Build history of the part. All positions in model axes, mm. Face numbers are marked on the shaded views. A direction names the side the tool comes from. Coordinates: 2 decimals unless noted, no trailing zeros. Loops run counter-clockwise (first coordinate to the right, second up) from the corner with the lowest first, then second, coordinate; pieces in that order, holes last.
(1) Slice it at D-D (x = -82.5). Give the cut face in (y, z).
(2) Flat gauge pins, fed straight in: P1, Ø6, axis at x = 1.5, z = -9.5, coming from the -Y side; P2, Ø1.5, axis at y = -232.5, z = -66.5, coming from the -X side; P3, Ø0.9, axis at y = -221.5, z = -13.5, coming from the +X side. Where does each tip first touch, or does it go through?
(3) Slice it at B-B (z = -96). Give the cut face in (x, y).
(4) Two-plate mould, pull along X, no slides. Class the marked faces 1, 2 and 3: pulls with the +X half, pulls with the -X half, needs draft (parallel to the pull), parting line crosses it, or undercut.
(5) Slice it at A-A (z = -12). Give the cut face in (x, y), and give its area (3 significant figures).
(6) Tool access for the marked faces 4 and 5: list every direction of +Z, -Z, +X, -X, +Y, -Y with a clear straight run to the whole face (end or side of a thin tool).
(7) Wall check: L1, parallel to Z at x = 0, y = -221; L2, parallel to X at y = -247, z = -1; L3, parallel to Y at x = 0, z = -1. Give the ranges that are in metal, low to high.
(8) Slice it at C-C (y = 102.5). Give the cut face in (x, z).
Autodesk Inventor part; units mm, degrees
ref_plane "Work Plane1" through (30, -275.6, -108.75) normal (1, 0, 0) x (0, 0, -1)
ref_plane "Work Plane2" through (0, -278.6, 0) normal (1, 0, 0) x (0, 0, -1)
ref_plane "Work Plane3" through (0, -275.6, 0) normal (1, 0, 0) x (0, 0, -1)
sketch "Sketch1" plane through (0, 0, 0) normal (0, 0, 1) x (1, 0, 0)
  line L0 (-100, 150) -> (100, 150)
  line L1 (100, 150) -> (100, -150)
  line L2 (-100, -150) -> (-100, 150)
  line L3 (-100, 150) -> (100, -150) construction
  line L4 (100, 150) -> (-100, -150) construction
  line L5 (100, -150) -> (36.4382, -213.5618)
  line L6 (-35.3571, -283.1536) -> (-35.3571, -323.1554)
  line L7 (-35.3571, -323.1554) -> (21.2114, -379.7239)
  line L8 (35.3571, -283.1536) -> (35.3571, -323.1554)
  line L9 (35.3571, -323.1554) -> (91.9257, -379.7239)
  line L10 (91.9257, -379.7239) -> (21.2114, -379.7239)
  arc A0 (-35.3571, -283.1536) -> (-35.3553, -283.1554) centre (0, -247.8) ccw
  arc A1 (-36.4382, -213.5618) -> (-35.3553, -283.1554) centre (0, -247.8) ccw
  arc A2 (35.3571, -283.1536) -> (36.4382, -213.5618) centre (0, -247.8) ccw
  line L11 (-100, -150) -> (-36.4382, -213.5618)
  point P0 (0, 0)
  point P1 (35.3571, -285.3571)
extrude "Extrusion1" add sketch "Sketch1" along normal blind 3
sketch "Sketch3" plane through (0, 0, 0) normal (0, 0, -1) x (-1, 0, 0)
  arc A0 (-36.4382, -213.5618) -> (-35.3571, -283.1536) centre (0, -247.8) ccw
  circle A1 centre (0, -247.8) radius 2.5
  circle A2 centre (0, -247.8) radius 4.75
  circle A3 centre (0, -247.8) radius 7.5
  point P0 (0, 0)
  dimension "d27" = 5
  dimension "d28" = 9.5
  dimension "d29" = 15
extrude "Extrusion4" cut sketch "Sketch3" against normal blind 3 contours A1
extrude "Extrusion5" add sketch "Sketch3" along normal blind 2 contours A3
sketch "Sketch4" plane through (0, 0, 0) normal (0, 0, -1) x (-1, 0, 0)
  line L0 (-30, -275.6) -> (30, -275.6)
  line L1 (30, -275.6) -> (30, -278.6)
  line L2 (30, -278.6) -> (-30, -278.6)
  line L3 (-30, -278.6) -> (-30, -275.6)
  line L4 (-30, -275.6) -> (30, -278.6) construction
  line L5 (30, -275.6) -> (-30, -278.6) construction
  circle A0 centre (0, -247.8) radius 2.5
  point P0 (0, 0)
  point P1 (0, -277.1)
  dimension "d34" = 60
  dimension "d35" = 3
  dimension "d36" = 27.8
extrude "Extrusion6" add sketch "Sketch4" along normal blind 108.75 contours L0 L1 L2 L3
ref_plane "Work Plane1" through (30, -275.6, -108.75) normal (1, 0, 0) x (0, 0, -1)
sketch "Sketch5" plane through (30, -275.6, -108.75) normal (1, 0, 0) x (0, 0, -1)
  line L0 (-108.75, 62.0382) -> (-108.75, -7.5536)
  line L1 (0, 0) -> (141.4214, 0) construction
  line L2 (-108.75, -47.5554) -> (-111.75, -47.5554)
  line L3 (-108.75, -3) -> (0, -3)
  line L4 (-108.75, -47.5554) -> (0, -3)
  line L5 (0, -3) -> (-108.75, -3)
  line L6 (-108.75, -3) -> (-108.75, -47.5554)
  point P0 (-108.75, 275.6)
  point P1 (-108.75, 0)
  point P2 (-108.75, 100)
ref_plane "Work Plane2" through (0, -278.6, 0) normal (1, 0, 0) x (0, 0, -1)
extrude "Extrusion8" add sketch "Sketch5" against normal blind 3
ref_plane "Work Plane3" through (0, -275.6, 0) normal (1, 0, 0) x (0, 0, -1)
mirror "Mirror2" about plane through (0, -275.6, 0) normal (1, 0, 0) of "Extrusion8"
sketch "Sketch6" plane through (0, 0, 0) normal (0, 0, -1) x (-1, 0, 0)
  line L0 (-15, -219.8) -> (15, -219.8)
  line L1 (15, -219.8) -> (15, -222.8)
  line L2 (15, -222.8) -> (-15, -222.8)
  line L3 (-15, -222.8) -> (-15, -219.8)
  line L4 (-15, -219.8) -> (15, -222.8) construction
  line L5 (15, -219.8) -> (-15, -222.8) construction
  circle A0 centre (0, -247.8) radius 2.5
  point P0 (0, 0)
  point P1 (0, -221.3)
  dimension "d46" = 30
  dimension "d47" = 3
  dimension "d48" = 25
extrude "Extrusion9" add sketch "Sketch6" along normal blind 40 contours L0 L1 L2 L3
sketch "Sketch7" plane through (-15, -219.8, 0) normal (0, 1, 0) x (1, 0, 0)
  circle A0 centre (15, 2.7) radius 1.5
  line L0 (115, 0) -> (-85, 0)
  line L1 (19, 6.2) -> (11, 6.2)
  line L2 (11, 6.2) -> (11, 18.2)
  line L3 (11, 18.2) -> (19, 18.2)
  line L4 (19, 18.2) -> (19, 6.2)
  line L5 (19, 6.2) -> (11, 18.2) construction
  line L6 (11, 6.2) -> (19, 18.2) construction
  circle A1 centre (15, 21.7) radius 1.5
  line L7 (21.5, 25.2) -> (0, 25.2)
  line L8 (1, 33.2) -> (21.5, 33.2)
  line L9 (21.5, 33.2) -> (21.5, 25.2)
  line L10 (21.5, 25.2) -> (8.5, 33.2) construction
  line L11 (8.5, 25.2) -> (21.5, 33.2) construction
  line L12 (1, 33.2) -> (0, 33.2)
  line L13 (0, 0) -> (0, 40)
  point P0 (15, 0)
  point P1 (15, 12.2)
  point P2 (15, 29.2)
  dimension "d51" = 3
  dimension "d52" = 2.7
  dimension "d53" = 8
  dimension "d54" = 12
  dimension "d55" = 3.5
  dimension "d56" = 3
  dimension "d57" = 3.5
  dimension "d60" = 3.5
extrude "Extrusion10" cut sketch "Sketch7" against normal mid plane 10
sketch "Sketch8" plane through (-30, -275.6, 0) normal (0, 1, 0) x (1, 0, 0)
  line L0 (0, 0) -> (0, 108.75)
  line L1 (0, 108.75) -> (60, 108.75)
  line L2 (60, 108.75) -> (60, 0)
  line L3 (60, 0) -> (0, 108.75) construction
  line L4 (0, 0) -> (60, 108.75) construction
  line L5 (57, 105.75) -> (3, 105.75)
  line L6 (3, 105.75) -> (3, 0)
  line L7 (57, 0) -> (57, 105.75)
  line L8 (60, 0) -> (57, 0)
  line L9 (3, 0) -> (0, 0)
  point P0 (30, 0)
  point P1 (30, 54.375)
extrude "Extrusion11" add sketch "Sketch8" along normal blind 62
sketch "Sketch9" plane through (-30, -213.6, 0) normal (0, 1, 0) x (1, 0, 0)
  line L0 (0, 0) -> (0, 108.75)
  line L1 (60, 0) -> (0, 0)
  line L2 (0, 0) -> (0, 108.75)
  line L3 (0, 108.75) -> (60, 108.75)
  line L4 (60, 108.75) -> (60, 0)
  point P0 (30, 0)
extrude "Extrusion12" add sketch "Sketch9" along normal blind 3
properties part number "rightside0"
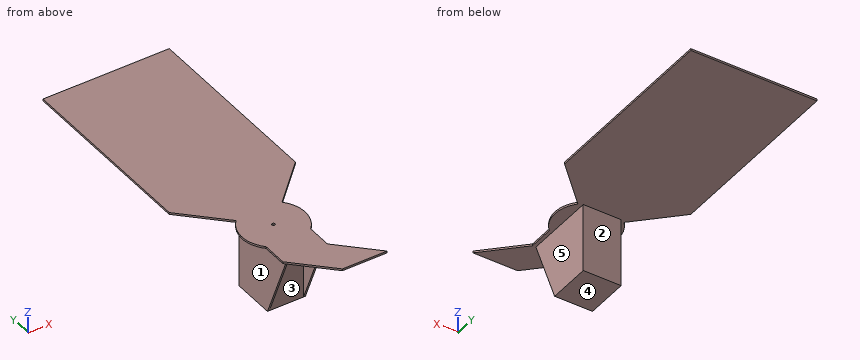
Response values:
1. outline: (-167.5, 0) - (150, 0) - (150, 3) - (-167.5, 3) - close
2. P1: stops at y = -278.6
2. P2: stops at x = -30
2. P3: stops at x = 30
3. outline: (-30, -283.82) - (-27, -283.82) - (-27, -278.6) - (27, -278.6) - (27, -283.82) - (30, -283.82) - (30, -210.6) - (-30, -210.6) - close; hole (-27, -275.6) - (27, -275.6) - (27, -213.6) - (-27, -213.6) - close
4. face 1: pulls with the -X half
4. face 2: needs draft
4. face 3: undercut
5. outline: (-30, -318.24) - (-27, -318.24) - (-27, -278.6) - (27, -278.6) - (27, -318.24) - (30, -318.24) - (30, -210.6) - (-30, -210.6) - close; (-15, -222.8) - (-4, -222.8) - (-4, -219.8) - (-15, -219.8) - close; (4, -222.8) - (15, -222.8) - (15, -219.8) - (4, -219.8) - close; hole (-27, -275.6) - (27, -275.6) - (27, -213.6) - (-27, -213.6) - close
5. area: 1,040 mm2
6. face 4: -Z, +X, -X, +Y, -Y
6. face 5: -Z, +X, +Y, -Y
7. L1: z = -108.75 to -105.75, -40 to -33.2, -25.2 to -23.2, -20.2 to -18.2, -6.2 to -4.2, -1.2 to 3
7. L2: x = -30 to -27, -7.46 to -4.68, 4.68 to 7.46, 27 to 30
7. L3: y = -278.6 to -275.6, -255.3 to -252.55, -243.05 to -240.3, -222.8 to -219.8, -213.6 to -210.6
8. outline: (-100, 0) - (100, 0) - (100, 3) - (-100, 3) - close
